from build123d import *

# Parameters (mm, degrees)
CHAFL_N1_SIZE         = 1
REDONDEO1_R           = 1
CHAFL_N2_SIZE         = 0.5
CROQUIS3_W            = 14.730869345
CROQUIS3_H            = 22.360679774
CORTAR_EXTRUIR1_DEPTH = 30
CHAFL_N3_SIZE         = 1
CHAFL_N3_SIZE2        = 1.12675647


with BuildPart() as part:
    # Croquis1 → Revolución1 (revolve)
    with BuildSketch(Plane.XY, mode=Mode.PRIVATE) as revoluci_n1_sk:
        Polygon((11.11, 48), (16, 48), (16, 30), (15, 30), (15, 20), (8.5, 20), (8.5, 17.951688966), (9, 17.951688966), (9, 0), (4.7625, 0), (4.7625, 32.24119236), (5.7625, 33.24119236), (9.525, 33.24119236), align=None)
    revolve(revoluci_n1_sk.sketch.rotate(Axis((0, 50.374990084, 0), (0, -1, 0)), 90), axis=Axis((0, 50.374990084, 0), (0, -1, 0)))

    # Chaflán1
    chafl_n1_edges = [part.edges().sort_by_distance(p)[0] for p in [
        (0, 0, -9),
    ]]
    chamfer(chafl_n1_edges, length=CHAFL_N1_SIZE)

    # Redondeo1
    # the kernel refuses this fillet: 1 mm, written as the material it takes off along each edge
    with BuildSketch(Plane(origin=(0, 17.951688966, 0), x_dir=(0, 0, 1), z_dir=(1, 0, 0))) as redondeo1_piece_1:
        with BuildLine():
            CenterArc((8, 0.866025404), REDONDEO1_R, 300, 60)
            Line((8.5, 0), (8.51, -0.017320508))
            ThreePointArc((8.51, -0.017320508), (8.75, -0.02), (9, -0.02))
            Line((9, -0.02), (9.02, 0))
            Line((9.02, 0), (9.02, 0.866025404))
            Line((9.02, 0.866025404), (9, 0.866025404))
        make_face()
    revolve(axis=Axis((0, 17.951688966, 0), (0, -1, 0)), mode=Mode.SUBTRACT)

    # Chaflán2
    chafl_n2_edges = [part.edges().sort_by_distance(p)[0] for p in [
        (0, 20, -15),
        (0, 30, -16),
        (0, 48, -16),
    ]]
    chamfer(chafl_n2_edges, length=CHAFL_N2_SIZE)

    # Croquis3 → Cortar-Extruir1 (cut)
    with BuildSketch(Plane.XZ):
        Polygon((10, 11.180339887), (10, -11.180339887), (24.245950338, -11.180339887), (24.827853146, 11.180339887), align=None)
        with Locations((-17.365434673, 0)):
            Rectangle(CROQUIS3_W, CROQUIS3_H)
    extrude(amount=-CORTAR_EXTRUIR1_DEPTH, mode=Mode.SUBTRACT)

    # Chaflán3
    chafl_n3_edges = [part.edges().sort_by_distance(p)[0] for p in [
        (0, 48, -11.11),
    ]]
    chafl_n3_side = [part.faces().sort_by_distance(p)[0] for p in [
        (0, 48, -15.061593796),
    ]]
    chamfer(chafl_n3_edges, length=CHAFL_N3_SIZE, length2=CHAFL_N3_SIZE2, reference=chafl_n3_side[0])


solid = part.part
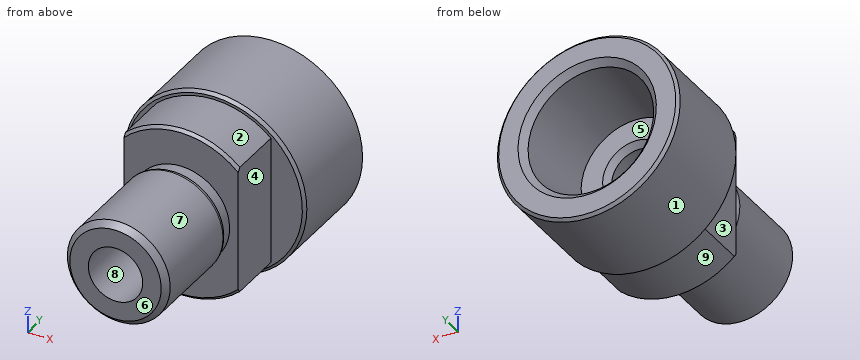
Read the model definition and answer for the solid it produces. Units are mm, in the model's axes. Face numbers are marked on the shaded views. A direction names the side the tool comes from. Coordinates: 2 decimals unless noted, no trailing zeros. Loops run counter-clockwise (first coordinate to the right, second up) from the corner with the lowest first, then second, coordinate; pieces in that order, holes last. Notation, with made-up numbers: (59.25, 61.5) -> (74.25, 61.5) arc R37 ccw to (74.25, 98.5) -> close; hole circle Ø9 at (64.5, -3.5). An arc over 180 degrees is marked (long way). Write item = value, one per line. Start each with the question number.
1) For the marked faces 1, 2, 3, 4 and 5, determine the directions among +Z, -Z, +X, -X, +Y, -Y from which every point of the face is accessible in a straight line to the end or side of a thin tool.
2) The part is cut by section C-C, the plane y = 39. Determine the outline of the cut face in (x, z), plus the area to 3 significant figures.
3) The mould has two halves that part along Z. Classify the marked faces 6, 7, 8 and 9: pulls with the +Z half, pulls with the -Z half, needs draft (parallel to the pull), parting line crosses it, or undercut.
4) The part is cut by section B-B, the plane y = 7. Determine the outline of the cut face in (x, z) (1 decimal), plus the area to 3 significant figures.
5) Given P1, Ø3, axis at x = 9, y = 6, coming from the +Z side; P2, Ø3, axis at x = 7.5, y = 32.5, coming from the +Z side; P3, Ø5, axis at y = 23, z = -2.5, coming from the -X side, each flat-ended and moving along its own axis, determine where each tip first touches the part or whether it passes through.
6) Find the intervals of material crossed by L1, parallel to X at y = 18.5, z = 0; L2, parallel to Y at x = 12, z = -7; L3, parallel to Y at x = 6, z = -13, in increasing order. Write a range as from..to.
Result:
q1.face_1 = +Y, -Y
q1.face_2 = +Z, -Y
q1.face_3 = +Z, -Z, -X, -Y
q1.face_4 = +Z, -Z, +X, -Y
q1.face_5 = +Y
q2.outline = circle Ø32 at (0, 0); hole circle Ø20.29 at (0, 0)
q2.area = 481 mm²
q3.face_6 = needs draft
q3.face_7 = parting line crosses it
q3.face_8 = undercut
q3.face_9 = pulls with the -Z half
q4.outline = circle Ø18 at (0, 0); hole circle Ø9.5 at (0, 0)
q4.area = 183 mm²
q5.P1 = 4.97
q5.P2 = 14.83
q5.P3 = -10
q6.L1 = -8.5..-4.76, 4.76..8.5
q6.L2 = 30..48
q6.L3 = 20..48
